The figure shows three views and two pictorial views of one solid part (mm, origin at its lowest corner). Answer the questions. A direction names the side the tool comes from. Coordinates: 2 decimals unless noted, no trailing zeros. Order: outer loops, then holes, each group sorted by start corner. A loop starts at its lowest first (then second) coordinate and runs counter-clockwise, first axis right, second up. Notation, with made-up numbers: M -6,78.25 L 0,78.25 A14 cw 0,102.25 Z; hole C -17.5,15 d6. An arc over 180 degrees is marked long. Answer in a Markdown table with one row per item. Add a question column.
Item 1: Which of the six approach directions +Z, -Z, +X, -X, +Y, -Y give full straight-line access (tool end or side, diameter ignored) to the marked faces 4 and 5?
Item 2: Consider line 1 (Z direction, x = 56, y = 6.5); line 2 (X direction, y = 9.75, z = 38); line 3 (X direction, y = 5, z = 10). Determine where each line is inside the solid, lowest interval first. Write a range as from..to.
Item 3: The part is cut by section C-C (z = 50). Write down the section's boundary in (x, y).
Item 4: The part is cut by section A-A (x = 50). Write down the section's boundary in (y, z), then the cut area to 3 significant figures.
Item 5: The part is cut by section D-D (z = 77). Write down the section's boundary in (x, y), then the cut area to 3 significant figures.
Item 6: The part is cut by section B-B (y = 1.5). Write down the section's boundary in (x, z).
Item 7: The mould has two halves that part along Z. Classify the marked faces 1, 2 and 3: released by +Z, released by -Z, zero draft, split by the parting line, or undercut.
Item 8: Flat-ended cylindrical pins translate along their axes: pin 1 Ø1.5 at (y, z) = (3, 53) entering from -X; pin 2 Ø5 at (y, z) = (5, 47.5) entering from -X; pin 3 Ø1.5 at (y, z) = (2, 75.5) entering from -X. Find the tip coordinate at first contact, or state that the pin passes through.
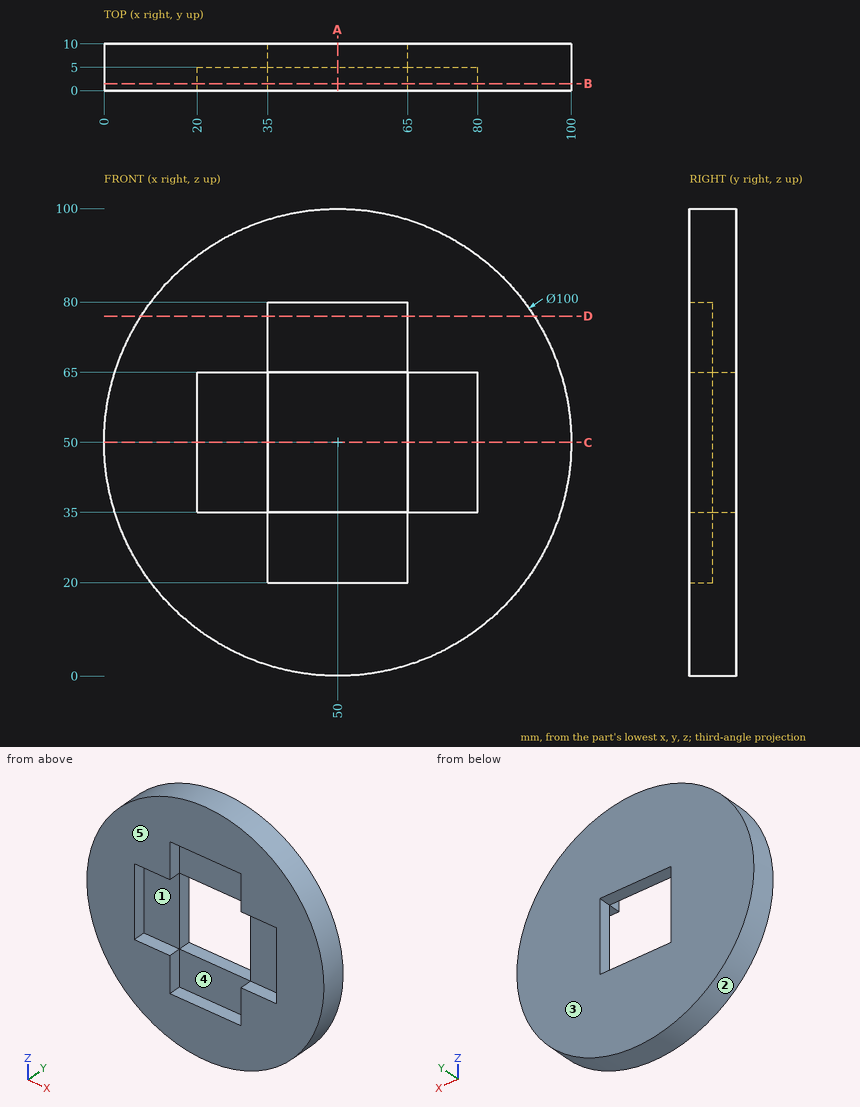
Reply:
| question | item | result |
|---|---|---|
| 1 | face 4 | -Y |
| 1 | face 5 | +Z, -Z, +X, -X, -Y |
| 2 | line 1 | z = 0.36..35, 65..99.64 |
| 2 | line 2 | x = 1.46..35, 65..98.54 |
| 2 | line 3 | x = 20..80 |
| 3 | outline | M 0,0 L 20,0 L 20,5 L 35,5 L 35,10 L 0,10 Z; M 65,5 L 80,5 L 80,0 L 100,0 L 100,10 L 65,10 Z |
| 4 | outline | M 0,0 L 10,0 L 10,35 L 5,35 L 5,20 L 0,20 Z; M 0,80 L 5,80 L 5,65 L 10,65 L 10,100 L 0,100 Z |
| 4 | area | 550 mm2 |
| 5 | outline | M 7.92,0 L 35,0 L 35,5 L 65,5 L 65,0 L 92.08,0 L 92.08,10 L 7.92,10 Z |
| 5 | area | 692 mm2 |
| 6 | outline | C 50,50 d100; hole M 20,35 L 35,35 L 35,20 L 65,20 L 65,35 L 80,35 L 80,65 L 65,65 L 65,80 L 35,80 L 35,65 L 20,65 Z |
| 7 | face 1 | undercut |
| 7 | face 2 | split by the parting line |
| 7 | face 3 | zero draft |
| 8 | pin 1 | stops at x = 0.05 |
| 8 | pin 2 | stops at x = 0 |
| 8 | pin 3 | stops at x = 6.56 |
